from build123d import *

# Parameters (mm, degrees)
SKETCH_3_R          = 9.6
EXTRUDE_1_DEPTH     = 8
CUT_EXTRUDE_3_DEPTH = 10
FILLET_1_R          = 10
CUT_EXTRUDE_4_DEPTH = 10


with BuildPart() as part:
    # 草图3 → 凸台-拉伸1 (new body)
    with BuildSketch(Plane(origin=(0, 0, 0), x_dir=(0, 0, -1), z_dir=(1, 0, 0))):
        with BuildLine():
            Line((14, -160), (14.949411629, -8.094139358))
            ThreePointArc((14.949411629, -8.094139358), (0, 17), (-14.949411629, -8.094139358))
            Line((-14.949411629, -8.094139358), (-14, -160))
            ThreePointArc((-14, -160), (0, -174), (14, -160))
        make_face()
        with Locations((0, -160)):
            Circle(SKETCH_3_R, mode=Mode.SUBTRACT)
    extrude(amount=EXTRUDE_1_DEPTH)

    # 草图6 → 切除-拉伸3 (cut)
    with BuildSketch(Plane(origin=(8, 0, 0), x_dir=(0, 0, -1), z_dir=(1, 0, 0))):
        with BuildLine():
            Line((5, -22.788825977), (5, -37.788825977))
            ThreePointArc((5, -37.788825977), (0, -42.788825977), (-5, -37.788825977))
            Line((-5, -37.788825977), (-5, -22.788825977))
            ThreePointArc((-5, -22.788825977), (0, -17.788825977), (5, -22.788825977))
        make_face()
        with BuildLine():
            Line((4.5, -54.788825977), (4.5, -74.788825977))
            ThreePointArc((4.5, -74.788825977), (0, -79.288825977), (-4.5, -74.788825977))
            Line((-4.5, -74.788825977), (-4.5, -54.788825977))
            ThreePointArc((-4.5, -54.788825977), (0, -50.288825977), (4.5, -54.788825977))
        make_face()
        with BuildLine():
            Line((4, -91.788825977), (4, -111.788825977))
            ThreePointArc((4, -111.788825977), (0, -115.788825977), (-4, -111.788825977))
            Line((-4, -111.788825977), (-4, -91.788825977))
            ThreePointArc((-4, -91.788825977), (0, -87.788825977), (4, -91.788825977))
        make_face()
        with BuildLine():
            Line((4, -128.788825977), (4, -138.788825977))
            ThreePointArc((4, -138.788825977), (0, -142.788825977), (-4, -138.788825977))
            Line((-4, -138.788825977), (-4, -128.788825977))
            ThreePointArc((-4, -128.788825977), (0, -124.788825977), (4, -128.788825977))
        make_face()
    extrude(amount=-CUT_EXTRUDE_3_DEPTH, mode=Mode.SUBTRACT)

    # 圆角1
    fillet_1_edges = [part.edges().sort_by_distance(p)[0] for p in [
        (4, -8.094139358, 14.949411629),
        (4, -8.094139358, -14.949411629),
    ]]
    fillet(fillet_1_edges, radius=FILLET_1_R)

    # 草图4 → 切除-拉伸4 (cut)
    with BuildSketch(Plane(origin=(8, 0, 0), x_dir=(0, 0, -1), z_dir=(1, 0, 0))):
        with BuildLine():
            Line((-3.071192312, 10.75), (-3.071192312, 9.095481174))
            ThreePointArc((-3.071192312, 9.095481174), (-8.313843876, 4.8), (-9.412513912, -1.888010025))
            Line((-9.412513912, -1.888010025), (-10.845369247, -2.715269438))
            ThreePointArc((-10.845369247, -2.715269438), (-11.969503653, -6.910596156), (-7.774176935, -8.034730562))
            Line((-7.774176935, -8.034730562), (-6.3413216, -7.207471149))
            ThreePointArc((-6.3413216, -7.207471149), (0, -9.6), (6.3413216, -7.207471149))
            Line((6.3413216, -7.207471149), (7.774176935, -8.034730562))
            ThreePointArc((7.774176935, -8.034730562), (11.969503653, -6.910596156), (10.845369247, -2.715269438))
            Line((10.845369247, -2.715269438), (9.412513912, -1.888010025))
            ThreePointArc((9.412513912, -1.888010025), (8.313843876, 4.8), (3.071192312, 9.095481174))
            Line((3.071192312, 9.095481174), (3.071192312, 10.75))
            ThreePointArc((3.071192312, 10.75), (0, 13.821192312), (-3.071192312, 10.75))
        make_face()
    extrude(amount=-CUT_EXTRUDE_4_DEPTH, mode=Mode.SUBTRACT)


solid = part.part
Read the model definition and answer for the solid it produces. Units are mm, in the model's axes. A direction names the side the tool comes from. Round coordinates to 2 decimals unless told otherwise and drop trailing zeros. Write each loop counter-clockwise with the first axis right and the second up, starting at its lowest first coordinate (ties: lowest second). Pieces come first, ordered by that corner, then holes.
1. The part is cut by section C-C, the plane y = -114. Determine the outline of the cut face in (x, z), then the cut area to 3 significant figures.
2. The part is cut by section A-A, the plane z = 0. Determine the outline of the cut face in (x, y).
3. Determine the mould class of faces 3 (the face through (4, -134, -4)), 4 (the face through (4.06, -8.4, -15.13)), 5 (the face through (0, -77.2, 4)), 6 (the face through (4.06, -87.79, 0.09)) for opening direction Z: pulls with the +Z half, pulls with the -Z half, needs draft (parallel to the pull), parting line crosses it, or undercut.
4. Straight lines are drawn through the part: L1, parallel to Y at x = 1.75, z = 6.5; L2, parallel to Y at x = 3, z = -5.5; L3, parallel to Z at x = 6.75, y = 4. For each, find the intervals that lie inside material, in ascending order.
5. Given pin 1 Ø4 at (x, y) = (5.5, -122.5) entering from -Z; pin 2 Ø3 at (x, z) = (5, -2) entering from -Y; pin 3 Ø2.5 at (x, y) = (5, -99) entering from +Z, each flat-ended and moving along its own axis, determine where each tip first touches the part or whether it passes through.
6. The part is cut by section B-B, the plane y = 0. Determine the outline of the cut face in (x, z).
7. Which of the six approach directions +Z, -Z, +X, -X, +Y, -Y give full straight-line access (tool end or side, diameter ignored) to faces 1 (the face through (4.06, -17.79, 0.11)), 2 (the face through (4.06, -8.34, 15.14))?
8. The part is cut by section D-D, the plane x = 2.75. State how many separate pieces and enclosed holes the cut face has, then the cut area to 3 significant figures.
Values:
1. outline: (0, -14.29) - (8, -14.29) - (8, -3.33) - (0, -3.33) - close; (0, 3.33) - (8, 3.33) - (8, 14.29) - (0, 14.29) - close
1. area: 175 mm2
2. outline: (0, -174) - (8, -174) - (8, -169.6) - (0, -169.6) - close; (0, -150.4) - (8, -150.4) - (8, -142.79) - (0, -142.79) - close; (0, -124.79) - (8, -124.79) - (8, -115.79) - (0, -115.79) - close; (0, -87.79) - (8, -87.79) - (8, -79.29) - (0, -79.29) - close; (0, -50.29) - (8, -50.29) - (8, -42.79) - (0, -42.79) - close; (0, -17.79) - (8, -17.79) - (8, -9.6) - (0, -9.6) - close; (0, 13.82) - (8, 13.82) - (8, 17) - (0, 17) - close
3. face 3: undercut
3. face 4: pulls with the -Z half
3. face 5: needs draft
3. face 6: undercut
4. L1: y = -172.4 to -167.06, -152.94 to -7.3, 7.06 to 15.71
4. L2: y = -172.87 to -167.87, -152.13 to -7.87, 7.87 to 16.09
4. L3: z = -16.52 to -8.73, 8.73 to 16.52
5. pin 1: stops at z = -14.25
5. pin 2: stops at y = -173.99
5. pin 3: stops at z = 14.39
6. outline: (0, -17) - (8, -17) - (8, -9.6) - (0, -9.6) - close; (0, 9.6) - (8, 9.6) - (8, 17) - (0, 17) - close
7. face 1: +X, -X
7. face 2: +Z, +X, -X, -Y
8. separate pieces: 1
8. enclosed holes: 6
8. area: 3,960 mm2
